Autodesk Inventor part; units mm, degrees
ref_plane "YZ Plane" through (0, 0, 0) normal (1, 0, 0) x (0, 1, 0)
ref_plane "XZ Plane" through (0, 0, 0) normal (0, 1, 0) x (-1, 0, 0)
ref_plane "XY Plane" through (0, 0, 0) normal (0, 0, 1) x (1, 0, 0)
sketch "草圖1" plane through (0, 0, 0) normal (0, 0, 1) x (1, 0, 0)
  line L0 (-50, 0) -> (0, 0) construction
  line L1 (-50, -5) -> (0, -5)
  line L2 (0, 5) -> (-50, 5)
  arc A0 (-50, 5) -> (-50, -5) centre (-50, 0) ccw
  arc A1 (0, -5) -> (0, 5) centre (0, 0) ccw
  circle A2 centre (-50, 0) radius 2.1
  circle A3 centre (0, 0) radius 2.1
  dimension "d0" = 50
  dimension "d1" = 10
  dimension "d2" = 4.2
  dimension "d3" = 4.2
extrude "擠出1" add sketch "草圖1" along normal blind 3
Model file for the job. Use its own axes, mm. Round coordinates to 2 decimals unless told otherwise and drop trailing zeros. Write each loop counter-clockwise with the first axis right and the second up, starting at its lowest first coordinate (ties: lowest second). Pieces come first, ordered by that corner, then holes. Notation, with made-up numbers: (13, -24.75) - (41, -24.75) arc R26 ccw to (41, -2.75) - close; hole circle Ø11 at (22.25, 52.25). An arc over 180 degrees is marked (long way). One line per item, written item: value.
(1) Wall check: probe 1 along Y at (x, z) = (0, 2.1); probe 2 along X at (y, z) = (-1.5, 2.6); probe 3 along X at (y, z) = (-1, 1.7). Give the ranges that are in metal, low to high.
Values follow:
probe 1: y = -5 to -2.1, 2.1 to 5
probe 2: x = -54.77 to -51.47, -48.53 to -1.47, 1.47 to 4.77
probe 3: x = -54.9 to -51.85, -48.15 to -1.85, 1.85 to 4.9
(2) Cut at A-A, the plane y = 0. Give the cut face in (x, z).
Values follow:
outline: (-55, 0) - (-52.1, 0) - (-52.1, 3) - (-55, 3) - close; (-47.9, 0) - (-2.1, 0) - (-2.1, 3) - (-47.9, 3) - close; (2.1, 0) - (5, 0) - (5, 3) - (2.1, 3) - close
(3) Two-plate mould, pull along X, no slides. Class faces 1 (the cylindrical face through (-48.06, 0.8, 1.48)), 2 (the cylindrical face through (-55, 0, 1)), 3 (the flat face through (-25, 0, 3)): pulls with the +X half, pulls with the -X half, needs draft (parallel to the pull), parting line crosses it, or undercut.
Values follow:
face 1: undercut
face 2: pulls with the -X half
face 3: needs draft
(4) Drop flat-ended pins along their axis: P1, Ø1, axis at y = -3.5, z = 1, coming from the +X side; P2, Ø3.5, axis at x = -50, y = 0, coming from the +Z side. Give the stop position or say it passes through.
Values follow:
P1: stops at x = 4
P2: passes through
(5) Cut at D-D, the plane y = -4.25. Give the cut face in (x, z), plus the area to 3 significant figures.
Values follow:
outline: (-52.63, 0) - (2.63, 0) - (2.63, 3) - (-52.63, 3) - close
area: 166 mm²
(6) Cut at B-B, the plane z = 1.15. Give the cut face in (x, y).
Values follow:
outline: (-50, -5) - (0, -5) arc R5 ccw to (0, 5) - (-50, 5) arc R5 ccw to start; hole circle Ø4.2 at (-50, 0); hole circle Ø4.2 at (0, 0)
(7) Cut at C-C, the plane y = 4. Give the cut face in (x, z).
Values follow:
outline: (-53, 0) - (3, 0) - (3, 3) - (-53, 3) - close
